```python
from build123d import *

# Parameters (mm, degrees)
CROQUIS1_R              = 115
SALIENTE_EXTRUIR1_DEPTH = 12
CROQUIS2_R              = 95
SALIENTE_EXTRUIR2_DEPTH = 140
CROQUIS3_R              = 4.7625
SALIENTE_EXTRUIR3_DEPTH = 10
MATRIZC1_COUNT          = 12
CROQUIS4_W              = 12.7
CROQUIS4_H              = 120
SALIENTE_EXTRUIR4_DEPTH = 100
CORTAR_EXTRUIR1_REACH   = 331.64
CROQUIS5_R              = 19.05
REDONDEO1_R             = 10


with BuildPart() as part:
    # Croquis1 → Saliente-Extruir1 (new body)
    with BuildSketch(Plane(origin=(0, 0, 0), x_dir=(1, 0, 0), z_dir=(0, 1, 0))):
        with Locations(Location((0, 0, 0), (0, 0, 270))):
            Circle(CROQUIS1_R)
    extrude(amount=SALIENTE_EXTRUIR1_DEPTH)

    # Croquis2 → Saliente-Extruir2 (add)
    with BuildSketch(Plane(origin=(0, 12, 0), x_dir=(1, 0, 0), z_dir=(0, 1, 0))):
        with Locations(Location((0, 0, 0), (0, 0, 270))):
            Circle(CROQUIS2_R)
    extrude(amount=SALIENTE_EXTRUIR2_DEPTH)

    # Croquis3 → Saliente-Extruir3 (add)
    with BuildSketch(Plane(origin=(0, 12, 0), x_dir=(1, 0, 0), z_dir=(0, 1, 0))):
        with Locations(Location((0, 105, 0), (0, 0, 270))):
            Circle(CROQUIS3_R)
    saliente_extruir3 = extrude(amount=SALIENTE_EXTRUIR3_DEPTH)

    # MatrizC1: Saliente-Extruir3 ×12 about axis
    matrizc1_axis = Axis((0, 0, 0), (0, 1, 0))
    for i in range(1, MATRIZC1_COUNT):
        add(saliente_extruir3.rotate(matrizc1_axis, i * 360 / MATRIZC1_COUNT))

    # Croquis4 → Saliente-Extruir4 (add)
    with BuildSketch(Plane(origin=(0, 152, 0), x_dir=(1, 0, 0), z_dir=(0, 1, 0))):
        with Locations((57.35, 0)):
            Rectangle(CROQUIS4_W, CROQUIS4_H)
        with Locations((-57.35, 0)):
            Rectangle(CROQUIS4_W, CROQUIS4_H)
    extrude(amount=SALIENTE_EXTRUIR4_DEPTH)

    # Cortar-Extruir1: up to this face of the body (flat: up to its plane)
    cortar_extruir1_end = Plane(part.part.faces().sort_by_distance((63.7, 202, 0))[0])
    # Croquis5 → Cortar-Extruir1 (cut, up to the picked face)
    with BuildSketch(Plane.ZY.offset(63.7), mode=Mode.PRIVATE) as cortar_extruir1_sk1:
        with Locations((0, 214)):
            Circle(CROQUIS5_R)
    cortar_extruir1_tool1 = split(extrude(cortar_extruir1_sk1.sketch, amount=-CORTAR_EXTRUIR1_REACH, mode=Mode.PRIVATE), bisect_by=cortar_extruir1_end, keep=Keep.BOTH, mode=Mode.PRIVATE)
    add(cortar_extruir1_tool1.solids().sort_by(Axis((-63.7, 214, 0), (1, 0, 0)))[0], mode=Mode.SUBTRACT)

    # Redondeo1
    redondeo1_edges = [part.edges().sort_by_distance(p)[0] for p in [
        (57.35, 252, 60),
        (57.35, 252, -60),
        (-57.35, 252, 60),
        (-57.35, 252, -60),
    ]]
    fillet(redondeo1_edges, radius=REDONDEO1_R)


solid = part.part
```
Geometry: final body of the model. Coordinates: model frame, mm. A direction names the side the tool comes from. Round coordinates to 2 decimals unless told otherwise and drop trailing zeros. Loops run counter-clockwise (first coordinate to the right, second up) from the corner with the lowest first, then second, coordinate; pieces in that order, holes last.
Item 1: Section B-B, the plane z = 0. State how many separate pieces and enclosed holes the cut face has, plus the area to 3 significant figures.
Checked values:
separate pieces: 3
enclosed holes: 0
area: 31,100 mm2
Item 2: Section A-A, the plane y = 189.5. Output: boundary loops of the cut face in (x, z), plus the area to 3 significant figures.
Checked values:
outline: (-63.7, -60) - (-51, -60) - (-51, 60) - (-63.7, 60) - close; (51, -60) - (63.7, -60) - (63.7, 60) - (51, 60) - close
area: 3,050 mm2
Item 3: Reachability of faces 1 (the flat face through (63.7, 190, 1)), 2 (the flat face through (-105, 22, 0)), 3 (the flat face through (0, 22, -105)) from +Z, -Z, +X, -X, +Y, -Y: full face, straight path, thin tool, end or side. Return the list, or none.
Checked values:
face 1: +Z, -Z, +X, +Y
face 2: +Z, -Z, -X, +Y
face 3: -Z, +X, -X, +Y
Item 4: Section C-C, the plane x = -105. Output: boundary loops of the cut face in (y, z).
Checked values:
outline: (0, -46.9) - (12, -46.9) - (12, -4.76) - (22, -4.76) - (22, 4.76) - (12, 4.76) - (12, 46.9) - (0, 46.9) - close
Item 5: Mould query, pull axis Z, two halves, no side actions, for faces 4 (the cylindrical face through (54.7, 16.93, -86.71)), 5 (the flat face through (57, 196, -60)), 6 (the cylindrical face through (-0.209, 16.93, 109.758)), 7 (the flat face through (91, 22, 53)). Classes: released by +Z, released by -Z, zero draft, split by the parting line, or undercut.
Checked values:
face 4: undercut
face 5: released by -Z
face 6: undercut
face 7: zero draft
Item 6: Line query: L1, parallel to Y at x = 56.25, z = 0; L2, parallel to Y at x = 16.5, z = 62; L3, parallel to X at y = 10, z = -0.5. Output: solid intervals per line, ascending.
Checked values:
L1: y = 0 to 194.95, 233.05 to 252
L2: y = 0 to 152
L3: x = -115 to 115
Item 7: Section D-D, the plane z = -28. Output: boundary loops of the cut face in (x, y).
Checked values:
outline: (-111.54, 0) - (111.54, 0) - (111.54, 12) - (90.78, 12) - (90.78, 152) - (63.7, 152) - (63.7, 252) - (51, 252) - (51, 152) - (-51, 152) - (-51, 252) - (-63.7, 252) - (-63.7, 152) - (-90.78, 152) - (-90.78, 12) - (-111.54, 12) - close
Item 8: Contact query for flat-ended pins moving along their axis: P1, Ø10.5, axis at x = -92, z = -54, coming from the +Y side; P2, Ø1, axis at x = 5.5, y = 114.5, coming from the -Z side; P3, Ø12, axis at y = 92, z = 25.5, coming from the +X side. Output: stop coordinate, or through.
Checked values:
P1: stops at y = 22
P2: stops at z = -94.87
P3: stops at x = 92.98
